Can you work these out from the model? Positions are in its coordinate system, mm. A direction names the side the tool comes from. Give positions to 0.01 mm unless a question says otherwise; leave off trailing zeros. Loops run counter-clockwise (first coordinate to the right, second up) from the corner with the lowest first, then second, coordinate; pieces in that order, holes last. Notation, with made-up numbers: M -34,2.5 L 12,2.5 A26 ccw 12,25.5 Z; hole C 9,79.5 d11. An arc over 180 degrees is marked long. Put each result on its own line as item: value. Start each with the question number.
1) Imagine slicing it at A-A (y = 0). Write out the boundary of the cut face in (x, z) (3 decimals), then the cut area to 3 significant figures.
2) If we mould it in two halves opening along X, with no side actions, what happens to faces 4 (the cylindrical face through (-6, 0, 2)), 5 (the flat face through (5, 0, 12.5)), 6 (the flat face through (19.772, -0.287, 3.451))? For each: +X half, -X half, draft (parallel to the pull), parting line (faces both ways), or undercut.
3) Please list where these lines run through material, in increasing order: line 1 along Y through (x, z) = (0, 1.6); line 2 along Y through (x, z) = (-3, 2.75); line 3 along Z through (x, y) = (5.5, -0.5). Write a range as from..to.
4) Imagine slicing it at B-B (x = 0). Write out the boundary of the cut face in (y, z), then the cut area to 4 significant figures.
5) Imagine slicing it at C-C (z = 2). Write out the boundary of the cut face in (x, y) (3 decimals).
6) For P1, Ø4, axis at x = 9, y = -3, coming from the -Z side; P2, Ø5, axis at y = -1.5, z = 8, coming from the -X side; P3, Ø4.5, axis at y = -7.5, z = 9, coming from the -X side; P4, Ø4.5, axis at y = -6, z = 11, coming from the +X side (3 decimals), each with a flat end and sliding along its axis, tell me the tip position at first contact or that it passes through.
7) For faces 1 (the flat face through (18.175, 0, 10)), 2 (the flat face through (-16.825, 0, 10)), 3 (the flat face through (3, 3, 4.5)), which set-ups out of +Z, -Z, +X, -X, +Y, -Y let a thin tool reach every point of the face, with its end or its side?
8) Imagine slicing it at D-D (y = -7). Write out the boundary of the cut face in (x, z) (3 decimals), then the cut area to 3 significant figures.
from build123d import *

# Parameters (mm, degrees)
F1_DEPTH       = 20.5
F3_D           = 6.5
F3_CBORE_D     = 12
F3_CBORE_DEPTH = 4.5
F4_DEPTH       = 5.5


with BuildPart() as f1:
    # F0 (on Front) → F1 (new body, symmetric)
    with BuildSketch(Plane.XZ):
        Polygon((-16.825, 7), (-21.325, 0), (21.325, 0), (18.175, 7), align=None)
    extrude(amount=F1_DEPTH, both=True)

    # F3 (through all)
    with Locations(Plane(origin=(0, 0, 0), x_dir=(1, 0, 0), z_dir=(0, 0, -1))):
        with Locations((0, 0)):
            CounterBoreHole(F3_D / 2, F3_CBORE_D / 2, F3_CBORE_DEPTH)

    # F4 (add): a face of the model
    f4_faces = [f1.faces().sort_by_distance(p)[0] for p in [
        (0.675, 19.9609267211, 7),
    ]]
    extrude(f4_faces, amount=F4_DEPTH)


solid = f1.part
Recorded:
1. outline: M -21.325,0 L -6,0 L -6,4.5 L -3.25,4.5 L -3.25,12.5 L -16.825,12.5 L -16.825,7 Z; M 3.25,4.5 L 6,4.5 L 6,0 L 21.325,0 L 18.175,7 L 18.175,12.5 L 3.25,12.5 Z
1. area: 358 mm²
2. face 4: undercut
2. face 5: draft
2. face 6: +X half
3. line 1: -20.5..-6, 6..20.5
3. line 2: -20.5..-5.2, 5.2..20.5
3. line 3: 4.5..12.5
4. outline: M -20.5,0 L -6,0 L -6,4.5 L -3.25,4.5 L -3.25,12.5 L -20.5,12.5 Z; M 3.25,4.5 L 6,4.5 L 6,0 L 20.5,0 L 20.5,12.5 L 3.25,12.5 Z
4. area: 406.5 mm²
5. outline: M -20.039,-20.5 L 20.425,-20.5 L 20.425,20.5 L -20.039,20.5 Z; hole C 0,0 d12
6. P1: z = 0
6. P2: x = -17.79
6. P3: x = -16.99
6. P4: x = 18.175
7. face 1: +Z, +X, +Y, -Y
7. face 2: +Z, -X, +Y, -Y
7. face 3: -Z
8. outline: M -21.325,0 L 21.325,0 L 18.175,7 L 18.175,12.5 L -16.825,12.5 L -16.825,7 Z
8. area: 464 mm²
